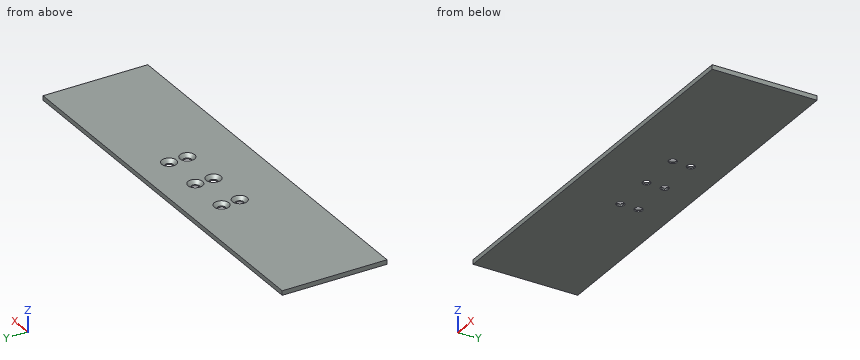
Autodesk Inventor part; units mm, degrees
ref_plane "YZ Plane" through (0, 0, 0) normal (1, 0, 0) x (0, 1, 0)
ref_plane "XZ Plane" through (0, 0, 0) normal (0, 1, 0) x (-1, 0, 0)
ref_plane "XY Plane" through (0, 0, 0) normal (0, 0, 1) x (1, 0, 0)
ref_plane "Work Plane1" through (0, 0, 0) normal (0, 0, 1) x (1, 0, 0)
sketch "Sketch1" plane through (0, 0, 0) normal (0, 0, 1) x (1, 0, 0)
  line L0 (0, 0) -> (47, 0)
  line L1 (47, 0) -> (47, 3)
  line L2 (0, 3) -> (47, 3)
  line L3 (0, 0) -> (0, 3)
  line L4 (-65.5, 38.5) -> (112.5, 38.5)
  line L5 (112.5, 38.5) -> (112.5, -8.5)
  line L6 (112.5, -8.5) -> (-65.5, -8.5)
  line L7 (-65.5, -8.5) -> (-65.5, 38.5)
  line L8 (-65, -11.5) -> (-65, 38.5)
  point P0 (23.5, 0)
  dimension "d0" = 178
  dimension "d1" = 89
  dimension "d2" = 89
  dimension "d3" = 0
  dimension "d13" = 3
extrude "Extrusion1" add sketch "Sketch1" along normal blind 2 contours L3 L2 L1 L0 | L4 L8 L6 L7 | L4 L5 L6 L8
sketch "Sketch2" plane through (0, 0, 2) normal (0, 0, 1) x (1, 0, 0)
  circle A0 centre (4, 23.825) radius 2.3
  circle A1 centre (4, 15.675) radius 2.3
  line L0 (7, 36.5) -> (1, 36.5)
  line L1 (1, 3) -> (1, 36.5)
  line L2 (1, 3) -> (7, 3)
  line L3 (7, 3) -> (7, 36.5)
  circle A2 centre (23.5, 23.825) radius 2.3
  circle A3 centre (23.5, 15.675) radius 2.3
  line L4 (28, 36.5) -> (19, 36.5)
  line L5 (19, 3) -> (19, 36.5)
  line L6 (19, 3) -> (28, 3)
  line L7 (28, 3) -> (28, 36.5)
  circle A4 centre (43, 23.825) radius 2.3
  circle A5 centre (43, 15.675) radius 2.3
  line L8 (46, 36.5) -> (40, 36.5)
  line L9 (40, 3) -> (40, 36.5)
  line L10 (40, 3) -> (46, 3)
  line L11 (46, 3) -> (46, 36.5)
  point P0 (0, 0)
hole "Hole1" at (4, 23.825, 2) at (4, 15.675, 2) at (23.5, 15.675, 2) at (23.5, 23.825, 2) at (43, 23.825, 2) at (43, 15.675, 2) direction (0, 0, -1) diameter 3.6 end through all countersink diameter 6.6 countersink angle 90
properties part number "back"
Model file for the job. Use its own axes, mm. Give positions to 0.01 mm unless a question says otherwise; leave off trailing zeros. Write each loop counter-clockwise with the first axis right and the second up, starting at its lowest first coordinate (ties: lowest second). Pieces come first, ordered by that corner, then holes. Notation, with made-up numbers: M 13.25,-20.5 L 61.25,-20.5 A19 ccw 61.25,-3.5 Z; hole C -33.5,38 d8. An arc over 180 degrees is marked long. Use a Markdown table: item, result.
1) Cut at B-B (z = 1.55). List the corners of the cut face in (x, y) (3 decimals).
Responses:
| item | result |
|---|---|
| outline | M -65.5,-8.5 L 112.5,-8.5 L 112.5,38.5 L -65.5,38.5 Z; hole C 4,15.675 d5.7; hole C 4,23.825 d5.7; hole C 23.5,15.675 d5.7; hole C 23.5,23.825 d5.7; hole C 43,15.675 d5.7; hole C 43,23.825 d5.7 |
2) Cut at A-A (x = 4). List the corners of the cut face in (y, z) (3 decimals).
Responses:
| item | result |
|---|---|
| outline | M -8.5,0 L 13.875,0 L 13.875,0.5 L 12.375,2 L -8.5,2 Z; M 17.475,0 L 22.025,0 L 22.025,0.5 L 20.525,2 L 18.975,2 L 17.475,0.5 Z; M 25.625,0 L 38.5,0 L 38.5,2 L 27.125,2 L 25.625,0.5 Z |
3) Pin check, flat tips, straight feed: pin 1 (4 mm diameter, centred on x = 43, y = 15.675, fed in from +Z); pin 2 (3 mm diameter, centred on x = 23.5, y = 23.825, fed in from +Z). Stop position of each tip, or through.
Responses:
| item | result |
|---|---|
| pin 1 | stops at z = 0.7 |
| pin 2 | passes through |
4) Drill centre lines: line 1 (Y direction, x = 23.5, z = 0.3) (3 decimals); line 2 (X direction, y = 22.5, z = 1.9); line 3 (X direction, y = 24.5, z = 1.05). Where is each one in solid material? Low to high. Write a range as from..to.
Responses:
| item | result |
|---|---|
| line 1 | y = -8.5..13.875, 17.475..22.025, 25.625..38.5 |
| line 2 | x = -65.5..1.09, 6.91..20.59, 26.41..40.09, 45.91..112.5 |
| line 3 | x = -65.5..1.75, 6.25..21.25, 25.75..40.75, 45.25..112.5 |
